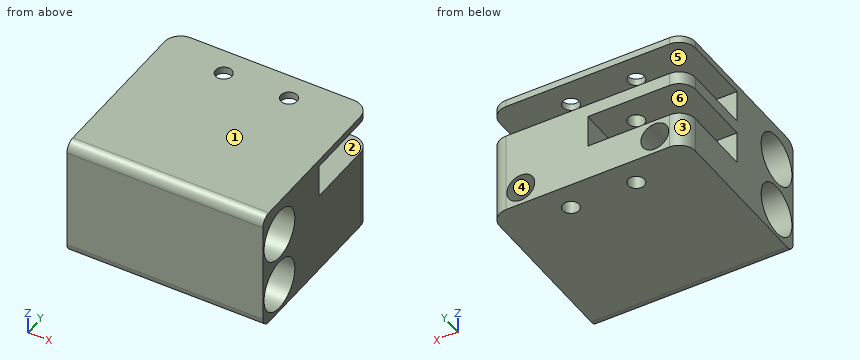
from build123d import *

# Parameters (mm, degrees)
RESSALTO_EXTRUS_O1_DEPTH = 40
ESBO_O4_R                = 7.8
CORTE_EXTRUS_O1_DEPTH    = 61
CORTE_EXTRUS_O2_DEPTH    = 3
FILETE2_R                = 3
CORTE_EXTRUS_O4_DEPTH    = 61
CORTE_EXTRUS_O5_DEPTH    = 30
ESBO_O10_R               = 2.5
CORTE_EXTRUS_O6_DEPTH    = 38
ESBO_O11_R               = 4.25
CORTE_EXTRUS_O7_DEPTH    = 30


with BuildPart() as part:
    # Esboço2 → Ressalto-extrusão1 (new body)
    with BuildSketch(Plane.XY):
        with BuildLine():
            Line((-246.218768802, 113.822486613), (-237.781231198, 113.822486613))
            Line((-237.781231198, 113.822486613), (-201.966801004, 113.822486613))
            Line((-201.966801004, 113.822486613), (-194.033198996, 113.822486613))
            Line((-194.033198996, 113.822486613), (-190, 113.822486613))
            Line((-190, 113.822486613), (-190, 138.123568891))
            Line((-190, 138.123568891), (-190, 163.212189341))
            ThreePointArc((-190, 163.212189341), (-191.464466094, 166.747723246), (-195, 168.212189341))
            Line((-195, 168.212189341), (-245, 168.212189341))
            ThreePointArc((-245, 168.212189341), (-248.535533906, 166.747723246), (-250, 163.212189341))
            Line((-250, 163.212189341), (-250, 138.123568891))
            Line((-250, 138.123568891), (-250, 113.822486613))
            Line((-250, 113.822486613), (-246.218768802, 113.822486613))
        make_face()
    extrude(amount=RESSALTO_EXTRUS_O1_DEPTH)

    # Esboço4 → Corte-extrusão1 (cut, through all)
    with BuildSketch(Plane(origin=(-190, 0, 0), x_dir=(0, 0, -1), z_dir=(1, 0, 0))):
        with Locations((-11.90241208, 122.212171493)):
            Circle(ESBO_O4_R)
        with Locations((-28.90241208, 122.212171493)):
            Circle(ESBO_O4_R)
    extrude(amount=-CORTE_EXTRUS_O1_DEPTH, mode=Mode.SUBTRACT)

    # Esboço5 → Corte-extrusão2 (cut)
    with BuildSketch(Plane(origin=(0, 0, 0), x_dir=(-1, 0, 0), z_dir=(0, 0, -1))):
        with BuildLine():
            Line((190, 163.212189341), (190, 113.822486613))
            Line((190, 113.822486613), (250, 113.822486613))
            Line((250, 113.822486613), (250, 163.212189341))
            ThreePointArc((250, 163.212189341), (248.535533906, 166.747723246), (245, 168.212189341))
            Line((245, 168.212189341), (195, 168.212189341))
            ThreePointArc((195, 168.212189341), (191.464466094, 166.747723246), (190, 163.212189341))
        make_face()
    extrude(amount=-CORTE_EXTRUS_O2_DEPTH, mode=Mode.SUBTRACT)

    # Filete2
    filete2_edges = [part.edges().sort_by_distance(p)[0] for p in [
        (-220, 113.822486613, 40),
        (-220, 113.822486613, 3),
    ]]
    fillet(filete2_edges, radius=FILETE2_R)

    # Esboço7 → Corte-extrusão4 (cut, through all)
    with BuildSketch(Plane(origin=(-190, 0, 0), x_dir=(0, 0, -1), z_dir=(1, 0, 0))):
        Polygon((-37.874860756, 142.212171493), (-37.874860756, 152.212171493), (-37.874860756, 170.639409053), (-27.874860756, 170.639409053), (-27.874860756, 152.212171493), (-27.874860756, 142.212171493), align=None)
    extrude(amount=-CORTE_EXTRUS_O4_DEPTH, mode=Mode.SUBTRACT)

    # Esboço8 → Corte-extrusão5 (cut)
    with BuildSketch(Plane.ZY.offset(250)):
        Polygon((23.874860756, 142.212171493), (23.874860756, 152.212171493), (23.874860756, 182.191519565), (13.874860756, 182.191519565), (13.874860756, 152.212171493), (13.874860756, 142.212171493), align=None)
    extrude(amount=-CORTE_EXTRUS_O5_DEPTH, mode=Mode.SUBTRACT)

    # Esboço10 → Corte-extrusão6 (cut, through all)
    with BuildSketch(Plane.XY.offset(40)):
        with Locations((-210, 160.173107934)):
            Circle(ESBO_O10_R)
        with Locations((-230, 160.173107934)):
            Circle(ESBO_O10_R)
    extrude(amount=-CORTE_EXTRUS_O6_DEPTH, mode=Mode.SUBTRACT)

    # Esboço11 → Corte-extrusão7 (cut)
    with BuildSketch(Plane(origin=(0, 168.212189341, 0), x_dir=(1, 0, 0), z_dir=(0, 1, 0))):
        with Locations((-199.5, -8.5)):
            Circle(ESBO_O11_R)
        with Locations((-240.5, -8.5)):
            Circle(ESBO_O11_R)
    extrude(amount=-CORTE_EXTRUS_O7_DEPTH, mode=Mode.SUBTRACT)


solid = part.part
The model under review builds one solid part; all positions refer to its coordinate system, in mm. Face numbers are marked on the shaded views. A direction names the side the tool comes from. Round coordinates to 2 decimals unless told otherwise and drop trailing zeros. Order: outer loops, then holes, each group sorted by start corner. A loop starts at its lowest first (then second) coordinate and runs counter-clockwise, first axis right, second up. Notation, with made-up numbers: (53.5, -38.5) -> (68.5, -38.5) arc R22 cw to (68.5, -16.5) -> close; hole circle Ø9 at (36.5, 52.5). An arc over 180 degrees is marked (long way). Write item = value, one per line. Start each with the question number.
Item 1: Consider section B-B on x = -210. Write out the cut boundary in (y, z).
Item 2: Mouldability with a two-part tool opening along Z and no side actions: class the marked faces 1, 2 and 3 as released by +Z, released by -Z, zero draft, split by the parting line, or undercut.
Item 3: Consider section C-C on y = 127. Write out the cut boundary in (x, z).
Item 4: For the marked faces 4, 5 and 6, list the 3-axis set-ups (+Z, -Z, +X, -X, +Y, -Y) from which the entire face can be reached by the end or side of a thin tool; tool diameter is ignored.
Item 5: Clearance check with flat-ended pins moving along their axes: pin 1 Ø4 at (x, z) = (-201.5, 7) entering from +Y; pin 2 Ø9.5 at (y, z) = (122.21, 11.9) entering from -X (3 decimals); pin 3 Ø8 at (y, z) = (161, 18) entering from -X. State where each tip first meets the part, or that it passes through.
Item 6: For line 1 along Z through (x, y) = (-225, 145.5); line 2 along X through (y, z) = (148, 8.5); line 3 along Z through (x, y) = (-231, 116.5), list the stretches that pass through material, from the lowest coordinate up.
Item 7: Consider section D-D on z = 18. Write out the cut boundary in (x, y).
Item 8: Consider section A-A on z = 12. Write out the cut boundary in (x, y), plus the area to 3 significant figures.
Conclusion:
q1.outline = (113.82, 6) arc R3 ccw to (116.82, 3) -> (157.67, 3) -> (157.67, 27.87) -> (142.21, 27.87) -> (142.21, 37.87) -> (157.67, 37.87) -> (157.67, 40) -> (116.82, 40) arc R3 ccw to (113.82, 37) -> close; (162.67, 3) -> (168.21, 3) -> (168.21, 27.87) -> (162.67, 27.87) -> close; (162.67, 37.87) -> (168.21, 37.87) -> (168.21, 40) -> (162.67, 40) -> close; hole circle Ø15.6 at (122.21, 11.9); hole circle Ø15.6 at (122.21, 28.9)
q2.face_1 = released by +Z
q2.face_2 = undercut
q2.face_3 = zero draft
q3.outline = (-250, 3) -> (-190, 3) -> (-190, 5.74) -> (-250, 5.74) -> close; (-250, 18.06) -> (-190, 18.06) -> (-190, 22.74) -> (-250, 22.74) -> close; (-250, 35.06) -> (-190, 35.06) -> (-190, 40) -> (-250, 40) -> close
q4.face_4 = +Y
q4.face_5 = +X, -X, +Y
q4.face_6 = -X, +Y
q5.pin_1 = 168.21
q5.pin_2 = through
q5.pin_3 = -220
q6.line_1 = 3 to 13.87, 23.87 to 27.87, 37.87 to 40
q6.line_2 = -250 to -244.75, -236.25 to -203.75, -195.25 to -190
q6.line_3 = 3.02 to 6.59, 17.21 to 23.59, 34.21 to 39.98
q7.outline = (-250, 113.82) -> (-190, 113.82) -> (-190, 117.35) -> (-250, 117.35) -> close; (-250, 127.08) -> (-190, 127.08) -> (-190, 163.21) arc R5 ccw to (-195, 168.21) -> (-220, 168.21) -> (-220, 142.21) -> (-250, 142.21) -> close; hole circle Ø5 at (-210, 160.17)
q8.outline = (-250, 113.82) -> (-190, 113.82) -> (-190, 114.41) -> (-250, 114.41) -> close; (-250, 130.01) -> (-190, 130.01) -> (-190, 163.21) arc R5 ccw to (-195, 168.21) -> (-197.09, 168.21) -> (-197.09, 138.21) -> (-201.91, 138.21) -> (-201.91, 168.21) -> (-238.09, 168.21) -> (-238.09, 138.21) -> (-242.91, 138.21) -> (-242.91, 168.21) -> (-245, 168.21) arc R5 ccw to (-250, 163.21) -> close; hole circle Ø5 at (-230, 160.17); hole circle Ø5 at (-210, 160.17)
q8.area = 1,990 mm2
